Model file for the job. Use its own axes, mm. A direction names the side the tool comes from. Coordinates: 2 decimals unless noted, no trailing zeros. Order: outer loops, then holes, each group sorted by start corner. A loop starts at its lowest first (then second) coordinate and runs counter-clockwise, first axis right, second up. Notation, with made-up numbers: M 53,79 L 93,79 A34 cw 93,110 Z; hole C -34.75,24 d5. An arc over 180 degrees is marked long. Return JSON: item names as keys, results as strings.
```python
from build123d import *

# Parameters (mm, degrees)
CUT_EXTRUDE1_DEPTH      = 391.541482324
CUT_EXTRUDE1_DEPTH_BACK = 391.541482324
SKETCH6_W               = 140
SKETCH6_H               = 298.689117204


with BuildPart() as part:
    # Sketch1 → Revolve1 (revolve)
    with BuildSketch(Plane.XY, mode=Mode.PRIVATE) as revolve1_sk:
        with BuildLine():
            Line((192.877031349, 42.655012217), (215.127149697, 29.808876046))
            ThreePointArc((215.127149697, 29.808876046), (224.106622413, 26.089455548), (233.742783423, 24.820826336))
            ThreePointArc((233.742783423, 24.820826336), (235.713203517, 25.027826984), (237.597587303, 25.639792966))
            add(Edge.make_bspline(
                [(237.597587303, 25.639792966), (305.794911856, 55.987196879), (370.436287167, 74.957098261)],
                knots=[0, 0, 0, 1, 1, 1], degree=2))
            Line((370.436287167, 74.957098261), (370.436287167, 87.463153647))
            Line((370.436287167, 87.463153647), (367.057221516, 86.471520319))
            add(Edge.make_bspline(
                [(233.22019623, 36.826239285), (236.069082049, 38.09248657), (241.789514517, 40.609481325), (253.162518773, 45.510982188), (267.324585603, 51.421835133), (284.209562024, 58.15884205), (300.991410001, 64.542388321), (317.668219236, 70.571409981), (334.241993713, 76.246293785), (347.963085648, 80.678672393), (358.895885037, 84.049397838), (364.330437681, 85.671308068), (367.057221516, 86.471520319)],
                knots=[0.492865274, 0.492865274, 0.492865274, 0.492865274, 0.492972774, 0.493080274, 0.493295274, 0.493510274, 0.493725274, 0.493940275, 0.494155275, 0.494370275, 0.494477775, 0.494585275, 0.494585275, 0.494585275, 0.494585275], degree=3))
            ThreePointArc((233.22019623, 36.826239285), (226.960399594, 37.749503395), (221.127153585, 40.201178647))
            Line((221.127153585, 40.201178647), (198.877039879, 53.047312137))
            ThreePointArc((198.877039879, 53.047312137), (172.857293904, 63.825067551), (144.9346606, 67.5011717))
            Line((144.9346606, 67.5011717), (0, 67.5011717))
            Line((0, 67.5011717), (0, 55.5011717))
            Line((0, 55.5011717), (144.9346606, 55.5011717))
            ThreePointArc((144.9346606, 55.5011717), (169.751460606, 52.23395891), (192.877031349, 42.655012217))
        make_face()
    revolve(revolve1_sk.sketch.rotate(Axis((0, 0, 0), (1, 0, 0)), 90), axis=Axis((0, 0, 0), (1, 0, 0)))

    # Sketch6 → Cut-Extrude1 (cut, two sides: drawn at the far end of the back side and taken through both)
    with BuildSketch(Plane.XY.offset(-CUT_EXTRUDE1_DEPTH_BACK)):
        with Locations((360.486, 0)):
            Rectangle(SKETCH6_W, SKETCH6_H)
    extrude(amount=CUT_EXTRUDE1_DEPTH + CUT_EXTRUDE1_DEPTH_BACK, mode=Mode.SUBTRACT)


solid = part.part
```
Item 1: Pull direction Y, two halves, no side cores. Call faces 1 (the flat face through (0, 55, -10)), 2 (the conical face through (219.735, 40.03, -8.889)), 3 (the conical face through (214.05, 27, 14.04)): +Y half, -Y half, draft (parallel to the pull), parting line (faces both ways), or undercut.
Check result:
{"face 1": "draft", "face 2": "parting line", "face 3": "undercut"}
Item 2: Drop flat-ended pins along their axis: pin 1 Ø3 at (x, z) = (260.5, 3) entering from +Y; pin 2 Ø1 at (x, y) = (240.5, 34.5) entering from -Z; pin 3 Ø6 at (x, y) = (75.5, -14.5) entering from +Z. Give the stop position or say it passes through.
Check result:
{"pin 1": "stops at y = 49.1", "pin 2": "stops at z = -21.24", "pin 3": "stops at z = 66.51"}
Item 3: Wall check: line 1 (Y direction, x = 115, z = 0); line 2 (Y direction, x = 146.5, z = 1.5); line 3 (Z direction, x = 46.5, y = -16). Give the ranges that are in metal, low to high.
Check result:
{"line 1": "y = -67.5 to -55.5, 55.5 to 67.5", "line 2": "y = -67.47 to -55.47, 55.47 to 67.47", "line 3": "z = -65.58 to -53.14, 53.14 to 65.58"}
Item 4: Saw through at A-A (x = 129). Write the cut outline in (y, z), and give its area (3 significant figures).
Check result:
{"outline": "C 0,0 d135; hole C 0,0 d111", "area": "4,640 mm2"}
Item 5: 3-axis set-ups, long thin cutter, end or side, ignore diameter. For faces 4 (the cylindrical face through (73.48, 49.24, 25.61)), 5 (the cylindrical face through (71.453, 65.896, -14.633)): which of +Z, -Z, +X, -X, +Y, -Y reach the whole face in a straight line?
Check result:
{"face 4": "-X", "face 5": "+X, -X"}
